Design review of the part shown in the three views and the two pictorial views. Dimensions are in mm from the part's minimum x, y and z. A direction names the side the tool comes from. Coordinates: 2 decimals unless noted, no trailing zeros. Order: outer loops, then holes, each group sorted by start corner. A loop starts at its lowest first (then second) coordinate and runs counter-clockwise, first axis right, second up. Notation, with made-up numbers: M -39.5,54.5 L -26.5,54.5 A27 cw -26.5,92.5 Z; hole C -16,60.25 d9. An arc over 180 degrees is marked long. Use CSV: the item, a comma, the result in double quotes.
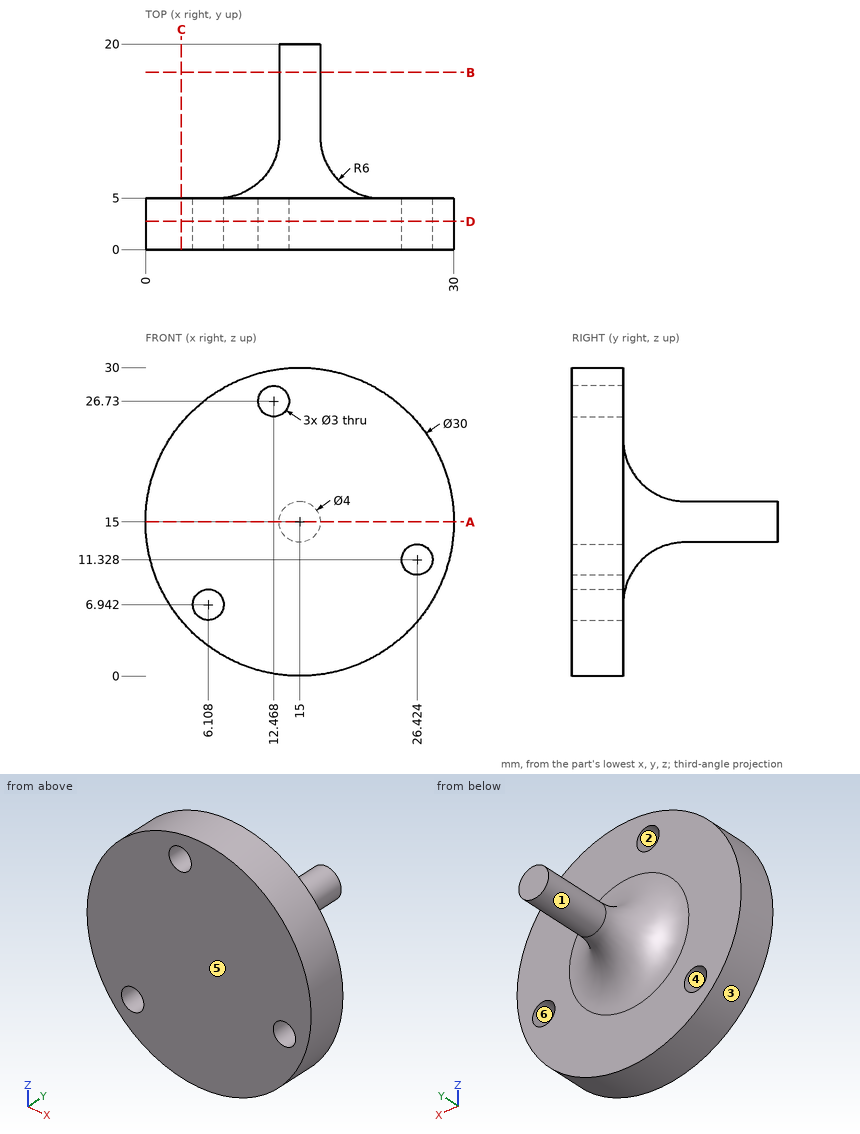
(1) Add section C-C on x = 3.5. State the section outline as (y, z) points, and give its area (3 significant figures).
The answers:
outline,"M 0,5.37 L 5,5.37 L 5,24.63 L 0,24.63 Z"
area,"96.3 mm2"
(2) Add section D-D on y = 2.75. State the section outline as (x, z) points (1 decimal), and give its area (3 significant figures).
The answers:
outline,"C 15,15 d30; hole C 6.1,6.9 d3; hole C 12.5,26.7 d3; hole C 26.4,11.3 d3"
area,"686 mm2"
(3) The part is to be moulded in two halves that separate along X. For the marked faces 3, 4, 5 and 6, say which applies: pulls with the +X half, pulls with the -X half, needs draft (parallel to the pull), parting line crosses it, or undercut.
The answers:
face 3,"parting line crosses it"
face 4,"undercut"
face 5,"needs draft"
face 6,"undercut"
(4) For the marked faces 1 and 2, list the 3-axis set-ups (+Z, -Z, +X, -X, +Y, -Y) from which the entire face can be reached by the end or side of a thin tool; tool diameter is ignored.
The answers:
face 1,"+Y"
face 2,"+Y, -Y"
(5) Wall thickness on probe 1 along Y at (x, z) = (4.5, 9.5); probe 2 along X at (y, z) = (3.25, 3.75); probe 3 along Y at (x, z) = (13, 19.25): over which ranges is each line inside the solid? List them lowest first.
The answers:
probe 1,"y = 0 to 5"
probe 2,"x = 5.08 to 24.92"
probe 3,"y = 0 to 5.99"
(6) Add section A-A on z = 15. State the section outline as (x, y) points.
The answers:
outline,"M 0,0 L 30,0 L 30,5 L 23,5 A6 cw 17,11 L 17,20 L 13,20 L 13,11 A6 cw 7,5 L 0,5 Z"
(7) Clearance check with flat-ended pins moving along their axes: P1, Ø10, axis at x = 14, z = 8, coming from the -Y side; P2, Ø4, axis at x = 12.47, z = 26.73, coming from the +Y side; P3, Ø12, axis at x = 19, y = 17.5, coming from the -Z side; P4, Ø8, axis at x = 20, y = 14, coming from the +Z side. State where each tip first meets the part, or that it passes through.
The answers:
P1,"stops at y = 0"
P2,"stops at y = 5"
P3,"stops at z = 13"
P4,"stops at z = 16.73"
(8) Add section B-B on y = 17.25. State the section outline as (x, z) points, and give its area (3 significant figures).
The answers:
outline,"C 15,15 d4"
area,"12.6 mm2"
